Autodesk Inventor part; units mm, degrees
ref_plane "YZ Plane" through (0, 0, 0) normal (1, 0, 0) x (0, 1, 0)
ref_plane "XZ Plane" through (0, 0, 0) normal (0, 1, 0) x (-1, 0, 0)
ref_plane "XY Plane" through (0, 0, 0) normal (0, 0, 1) x (1, 0, 0)
sketch "Эскиз1" plane through (0, 0, 0) normal (0, 1, 0) x (-1, 0, 0)
  line L0 (0, 18) -> (0, -18)
  arc A0 (-57.1363, 7.7095) -> (-57.1363, -7.7095) centre (-55, 0) ccw
  line L1 (0, 0) -> (-6.25, 0) construction
  line L2 (0, 18) -> (-18.6401, 18)
  line L3 (-21.3105, 17.6369) -> (-57.1363, 7.7095)
  line L4 (0, -18) -> (-18.6401, -18)
  line L5 (-21.3105, -17.6369) -> (-57.1363, -7.7095)
  circle A1 centre (-55, 0) radius 2
  arc A2 (-18.6401, 18) -> (-21.3105, 17.6369) centre (-18.6401, 8) ccw
  arc A3 (-21.3105, -17.6369) -> (-18.6401, -18) centre (-18.6401, -8) ccw
  circle A4 centre (-10, -13) radius 1.75
  circle A5 centre (-10, 13) radius 1.75
  line L6 (-10, 13) -> (-10, -13) construction
  point P0 (-20, 18)
  dimension "d0" = 16
  dimension "d1" = 36
  dimension "d2" = 55
  dimension "d3" = 20
  dimension "d4" = 4
  dimension "d5" = 10
  dimension "d18" = 3.5
  dimension "d19" = 13
  dimension "d20" = 10
extrude "Выдавливание1" add sketch "Эскиз1" along normal blind 4
sketch "Эскиз2" plane through (0, 4, 0) normal (0, 1, 0) x (1, 0, 0)
  line L0 (0, 0) -> (14.985, 0) construction
  line L1 (0, 7.5) -> (22, 7.5)
  line L2 (22, 7.5) -> (22, -7.5)
  line L3 (22, -7.5) -> (0, -7.5)
  line L4 (0, -7.5) -> (0, 7.5)
  line L5 (0, 18) -> (0, -18)
  dimension "d8" = 15
  dimension "d9" = 22
extrude "Выдавливание2" add sketch "Эскиз2" along normal blind 2
chamfer "Фаска1" distance 2 angle 45 1 edges at (22, 6, 0)
chamfer "Фаска2" distance 0.5 angle 45 2 edges at (10.0002, 6, 7.5) (10.0003, 6, -7.5)
sketch "Эскиз4" plane through (0, 4, 0) normal (0, 1, 0) x (1, 0, 0)
  arc A0 (47.0304, -50.6972) -> (63, -50) centre (55, -50) ccw
  line L0 (63, -50) -> (63, 0)
  arc A1 (57.1363, -7.7095) -> (57.1363, 7.7095) centre (55, 0) ccw
  line L1 (47.0304, -50.6972) -> (43.5977, -11.461)
  line L2 (57.1363, -7.7095) -> (21.3105, -17.6369)
  circle A2 centre (55, -50) radius 4
  point P0 (0, 0)
  dimension "d21" = 16
  dimension "d22" = 50
  dimension "d23" = 55
  dimension "d24" = 5
  dimension "d34" = 8
  dimension "d35" = 55
extrude "Выдавливание3" add sketch "Эскиз4" against normal up to surface (4 mm away)
fillet "Сопряжение1" radius 10 1 edges at (43.5977, 2, 11.461)
sketch "Эскиз5" plane through (0, 4, 0) normal (0, 1, 0) x (1, 0, 0)
  circle A0 centre (55, 0) radius 2
  circle A1 centre (55, 0) radius 3
  point P0 (0, 0)
  dimension "d28" = 1
extrude "Выдавливание4" add sketch "Эскиз5" along normal blind 1
chamfer "Фаска3" distance 1 angle 45 1 edges at (52, 4, 0)
sketch "Эскиз7" plane through (0, 4, 0) normal (0, 1, 0) x (1, 0, 0)
  circle A0 centre (55, -50) radius 4
  circle A1 centre (55, -50) radius 5
  point P0 (0, 0)
  dimension "d36" = 10
extrude "Выдавливание5" cut sketch "Эскиз7" against normal blind 1
properties part number "04-06-Рычаг нижний"
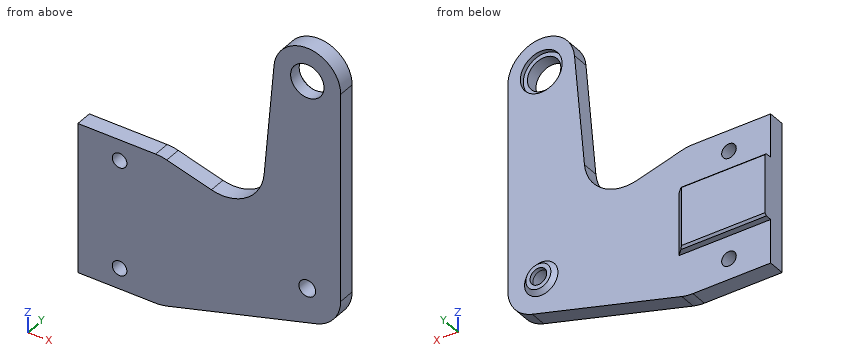
Geometry check sheet. Reference: the model listing, model coordinates, mm. Give positions to 0.01 mm unless a question says otherwise; leave off trailing zeros. Order: outer loops, then holes, each group sorted by start corner. A loop starts at its lowest first (then second) coordinate and runs counter-clockwise, first axis right, second up.
1. Sectioned sample at D-D (z = -13). Record the boundary of the cut face in (x, y), then the cut area to 3 significant figures.
Completed:
outline: (0, 0) - (8.25, 0) - (8.25, 4) - (0, 4) - close; (11.75, 0) - (38.04, 0) - (38.04, 4) - (11.75, 4) - close
area: 138 mm2
2. Scan lines: line 1 (Z direction, x = 10, y = 1); line 2 (Z direction, x = 55, y = 1.75); line 3 (X direction, y = 2.5, z = 27.5). Record each from-to range of solid material in increasing order.
Completed:
line 1: z = -18 to -14.75, -11.25 to 11.25, 14.75 to 18
line 2: z = -8.3 to -2, 2 to 46, 54 to 58
line 3: x = 45 to 63
3. Sectioned sample at B-B (z = 51.5). Record the boundary of the cut face in (x, y), then the cut area to 3 significant figures.
Completed:
outline: (47.14, 0) - (51.29, 0) - (51.29, 3) - (50.23, 3) - (50.23, 4) - (47.14, 4) - close; (58.71, 0) - (62.86, 0) - (62.86, 4) - (59.77, 4) - (59.77, 3) - (58.71, 3) - close
area: 31.1 mm2
4. Depth check by flat-ended pin: pin 1 (3 mm diameter, centred on x = 55, z = 0, fed in from -Y); pin 2 (2 mm diameter, centred on y = 1.5, z = 45.5, fed in from -X); pin 3 (6.5 mm diameter, centred on x = 55, z = 0, fed in from +Y); pin 4 (16 mm diameter, centred on x = 55, z = 50, fed in from -Y). Enter the tip coordinate at first touch or a pass-through.
Completed:
pin 1: passes through
pin 2: stops at x = 46.49
pin 3: stops at y = 5
pin 4: stops at y = 0
5. Sectioned sample at C-C (x = 55). State how many separate pieces and enclosed holes the cut face has, then the cut area to 3 significant figures.
Completed:
separate pieces: 3
enclosed holes: 0
area: 218 mm2
6. Sectioned sample at A-A (x = 10). Record the boundary of the cut face in (y, z), then the cut area to 3 significant figures.
Completed:
outline: (0, -18) - (4, -18) - (4, -14.75) - (0, -14.75) - close; (0, -11.25) - (4, -11.25) - (4, -7.5) - (5.5, -7.5) - (6, -7) - (6, 7) - (5.5, 7.5) - (4, 7.5) - (4, 11.25) - (0, 11.25) - close; (0, 14.75) - (4, 14.75) - (4, 18) - (0, 18) - close
area: 146 mm2
